Could you check a few things on this model? Use its own coordinates, in mm. A direction names the side the tool comes from. Coordinates: 2 decimals unless noted, no trailing zeros. Loops run counter-clockwise (first coordinate to the right, second up) from the corner with the lowest first, then second, coordinate; pieces in that order, holes last. Notation, with made-up numbers: (81, 31) - (126, 31) arc R25 ccw to (126, 66) - close; hole circle Ø8 at (25, 72.25). An arc over 180 degrees is marked (long way). Use CSV: the item, a comma, the result in double quotes.
from build123d import *

# Parameters (mm, degrees)
SKETCH2_R            = 15.4305
SKETCH2_R_2          = 2.0193
BOSS_EXTRUDE1_DEPTH  = 1.4
FILLET4_R            = 8.255
CUT_EXTRUDE1_DEPTH   = 2.4000001
FILLET5_R            = 8.89
FILLET5_OF_MIRROR1_R = 8.89
SKETCH8_R            = 4.5593
SKETCH8_R_2          = 2.0193
BOSS_EXTRUDE2_DEPTH  = 2.029


with BuildPart() as part:
    # Sketch2 → Boss-Extrude1 (new body)
    with BuildSketch(Plane.XY):
        with BuildLine():
            Line((-69.215, 12.7), (-69.215, 0))
            Line((-69.215, 0), (-62.357, 0))
            Line((-62.357, 0), (-62.357, 26.67))
            ThreePointArc((-62.357, 26.67), (-59.69, 29.337), (-57.023, 26.67))
            Line((-57.023, 26.67), (-57.023, 0))
            Line((-57.023, 0), (-50.165, 0))
            Line((-50.165, 0), (-50.165, 31.75))
            Line((-50.165, 31.75), (-19.05, 40.64))
            Line((-19.05, 40.64), (0, 40.64))
            Line((0, 40.64), (19.05, 40.64))
            Line((19.05, 40.64), (50.165, 31.75))
            Line((50.165, 31.75), (50.165, 0))
            Line((50.165, 0), (57.023, 0))
            Line((57.023, 0), (57.023, 26.67))
            ThreePointArc((57.023, 26.67), (59.69, 29.337), (62.357, 26.67))
            Line((62.357, 26.67), (62.357, 0))
            Line((62.357, 0), (69.215, 0))
            Line((69.215, 0), (69.215, 12.7))
            Line((69.215, 12.7), (69.215, 31.75))
            add(Edge.make_bspline(
                [(69.215, 31.75), (69.215, 54.201663529), (66.080158446, 63.077253183), (57.15, 82.55)],
                knots=[0, 0, 0, 0, 1, 1, 1, 1], degree=3))
            Line((57.15, 82.55), (-57.15, 82.55))
            add(Edge.make_bspline(
                [(-69.215, 31.75), (-69.215, 54.201663529), (-66.080158446, 63.077253183), (-57.15, 82.55)],
                knots=[0, 0, 0, 0, 1, 1, 1, 1], degree=3))
            Line((-69.215, 31.75), (-69.215, 12.7))
        make_face()
        with Locations((0, 62.742379961)):
            Circle(SKETCH2_R, mode=Mode.SUBTRACT)
        with Locations((-14.727620039, 48.014759923)):
            Circle(SKETCH2_R_2, mode=Mode.SUBTRACT)
        with Locations((14.727620039, 77.47)):
            Circle(SKETCH2_R_2, mode=Mode.SUBTRACT)
    extrude(amount=BOSS_EXTRUDE1_DEPTH)

    # Fillet4
    fillet4_edges = [part.edges().sort_by_distance(p)[0] for p in [
        (57.15, 82.55, 0.7),
        (-57.15, 82.55, 0.7),
        (50.165, 31.75, 0.7),
        (19.05, 40.64, 0.7),
        (-19.05, 40.64, 0.7),
        (-50.165, 31.75, 0.7),
    ]]
    fillet(fillet4_edges, radius=FILLET4_R)

    # Sketch7 → Cut-Extrude1 (cut, through all)
    with BuildSketch(Plane.XY.offset(1.4)):
        with BuildLine():
            Line((-22.501902321, 74.93), (-51.827314967, 74.93))
            Line((-51.827314967, 74.93), (-52.239495321, 74.93))
            Line((-52.239495321, 74.93), (-52.407305567, 74.553526409))
            add(Edge.make_bspline(
                [(-52.407305567, 74.553526409), (-53.292419845, 72.567818402), (-54.098016837, 70.709360728), (-55.558646263, 67.181996285), (-56.213641355, 65.513276159), (-57.386849267, 62.293765878), (-57.905181999, 60.743063744), (-58.823443884, 57.676179523), (-59.223597116, 56.159796082), (-59.922846669, 53.067471662), (-60.222031529, 51.491149103), (-60.491375272, 49.737636417), (-60.506543886, 49.637526891), (-60.521547991, 49.537125261)],
                knots=[0, 0, 0, 0, 0.125, 0.125, 0.25, 0.25, 0.375, 0.375, 0.5, 0.5, 0.625, 0.625, 0.632545784, 0.632545784, 0.632545784, 0.632545784], degree=3))
            ThreePointArc((-60.521547991, 49.537125261), (-57.650036676, 41.695346124), (-49.50226085, 39.864273665))
            Line((-49.50226085, 39.864273665), (-46.271197905, 40.787434507))
            Line((-46.271197905, 40.787434507), (-20.935753267, 48.026132975))
            ThreePointArc((-20.935753267, 48.026132975), (-25.547250262, 61.255203349), (-22.501902321, 74.93))
        make_face()
    cut_extrude1 = extrude(amount=-CUT_EXTRUDE1_DEPTH, mode=Mode.SUBTRACT)

    # Fillet5
    fillet5_edges = [part.edges().sort_by_distance(p)[0] for p in [
        (-22.501902321, 74.93, 0.7),
        (-52.239495321, 74.93, 0.7),
        (-20.935753267, 48.026132975, 0.7),
    ]]
    fillet(fillet5_edges, radius=FILLET5_R)

    # Mirror1: Cut-Extrude1 across plane
    add(cut_extrude1.mirror(Plane(origin=(0, 0, 0), x_dir=(0, 0, 1), z_dir=(1, 0, 0))), mode=Mode.SUBTRACT)

    # Fillet5 of Mirror1
    fillet5_of_mirror1_edges = [part.edges().sort_by_distance(p)[0] for p in [
        (22.501902321, 74.93, 0.7),
        (52.239495321, 74.93, 0.7),
        (20.935753267, 48.026132975, 0.7),
    ]]
    fillet(fillet5_of_mirror1_edges, radius=FILLET5_OF_MIRROR1_R)

    # Sketch8 → Boss-Extrude2 (add)
    with BuildSketch(Plane(origin=(0, 0, 0), x_dir=(-1, 0, 0), z_dir=(0, 0, -1))):
        with Locations((-14.727620039, 77.47)):
            Circle(SKETCH8_R)
        with Locations((-14.727620039, 77.47)):
            Circle(SKETCH8_R_2, mode=Mode.SUBTRACT)
        with Locations((14.727620039, 48.014759923)):
            Circle(SKETCH8_R)
        with Locations((14.727620039, 48.014759923)):
            Circle(SKETCH8_R_2, mode=Mode.SUBTRACT)
    extrude(amount=BOSS_EXTRUDE2_DEPTH)


solid = part.part
(1) Suppose I cut it at A-A (y = 9.5). Write out the boundary of the cut face in (x, z) (3 decimals), plus the area to 3 significant figures.
Computed:
outline,"(-69.215, 0) - (-62.357, 0) - (-62.357, 1.4) - (-69.215, 1.4) - close; (-57.023, 0) - (-50.165, 0) - (-50.165, 1.4) - (-57.023, 1.4) - close; (50.165, 0) - (57.023, 0) - (57.023, 1.4) - (50.165, 1.4) - close; (62.357, 0) - (69.215, 0) - (69.215, 1.4) - (62.357, 1.4) - close"
area,"38.4 mm²"
(2) Suppose I cut it at B-B (x = 0). Write out the boundary of the cut face in (y, z).
Computed:
outline,"(40.64, 0) - (47.31, 0) - (47.31, 1.4) - (40.64, 1.4) - close; (78.17, 0) - (82.55, 0) - (82.55, 1.4) - (78.17, 1.4) - close"
(3) Please list where these lines run through material, in increasing order: line 1 (X direction, y = 3, z = 0.35) (3 decimals); line 2 (Z direction, x = 62, y = 42.5); line 3 (X direction, y = 65, z = 0.9).
Computed:
line 1,"x = -69.215 to -62.357, -57.023 to -50.165, 50.165 to 57.023, 62.357 to 69.215"
line 2,"z = 0 to 1.4"
line 3,"x = -64.5 to -56.39, -25.49 to -15.26, 15.26 to 25.49, 56.39 to 64.5"
(4) Suppose I cut it at D-D (x = 33). Write out the boundary of the cut face in (y, z).
Computed:
outline,"(36.65, 0) - (44.58, 0) - (44.58, 1.4) - (36.65, 1.4) - close; (74.83, 0) - (82.55, 0) - (82.55, 1.4) - (74.83, 1.4) - close"
(5) Suppose I cut it at C-C (z = -1). Write out the boundary of the cut face in (x, y).
Computed:
outline,"circle Ø9.12 at (-14.73, 48.01); circle Ø9.12 at (14.73, 77.47); hole circle Ø4.04 at (-14.73, 48.01); hole circle Ø4.04 at (14.73, 77.47)"
(6) Will these pins go through, and if not, where does the flat tip stop? pin 1 (1 mm diameter, centred on x = 34, z = -1.5, fed in from +Y); pin 2 (1.5 mm diameter, centred on x = -38.5, z = 1, fed in from -Y); pin 3 (0.7 mm diameter, centred on x = 38.5, z = 1, fed in from -Y); pin 4 (12 mm diameter, centred on x = -15.5, y = 65, fed in from -Z).
Computed:
pin 1,"passes through"
pin 2,"stops at y = 34.87"
pin 3,"stops at y = 34.98"
pin 4,"stops at z = 0"
(7) Which directions (+Z, -Z, +X, -X, +Y, -Y) give clear straight access to the entire face, cutting with the end or side of a thin tool? Please do faces 4 (the face through (-48.55, 30.43, 0.71)), 5 (the face through (-16, 46, -2.029)), 6 (the face through (27.67, 71.94, 0.69)), 7 (the face through (-16, 51, 1.4)), 8 (the face through (15.32, 81.99, -1)).
Computed:
face 4,"+Z, -Z, -Y"
face 5,"-Z, +X, -X, +Y, -Y"
face 6,"+Z, -Z"
face 7,"+Z, +X, -X, +Y, -Y"
face 8,"-Z"
(8) Thinking about a two-plate mould opening in Y: for faces 1 (the face through (-14.134, 52.535, -1)), 2 (the face through (57.741, 41.776, 0.71)), 3 (the face through (59.631, 29.336, 0.69)), which applies, +Y half, -Y half, draft (parallel to the pull), parting line (faces both ways), or undercut?
Computed:
face 1,"parting line"
face 2,"undercut"
face 3,"-Y half"
